For this review, take the finished solid that the model builds, in its own axes (mm). A direction names the side the tool comes from. Round coordinates to 2 decimals unless told otherwise and drop trailing zeros. Write each loop counter-clockwise with the first axis right and the second up, starting at its lowest first coordinate (ties: lowest second). Pieces come first, ordered by that corner, then holes. Notation, with made-up numbers: (15.5, 45) - (51.5, 45) arc R24 cw to (51.5, 57) - close; hole circle Ø5 at (47.25, -8). An arc over 180 degrees is marked (long way). Answer in a Markdown table with one row per item. Add a question column.
from build123d import *

# Parameters (mm, degrees)
SKETCH2_W         = 80
SKETCH2_H         = 60
FLOOR_2P4_DEPTH   = 2.4
WALLS_2P4_START   = 2.4
SKETCH3_W         = 80
SKETCH3_H         = 60
SKETCH3_W_2       = 75.2
SKETCH3_H_2       = 55.2
WALLS_2P4_DEPTH   = 33.6
CATCH_LEFT_START  = 21
SKETCH4_W         = 0.8
SKETCH4_H         = 12
CATCH_LEFT_DEPTH  = 2
CATCH_RIGHT_START = 21
SKETCH5_W         = 0.8
SKETCH5_H         = 12
CATCH_RIGHT_DEPTH = 2


with BuildPart() as part:
    # Sketch2 → Floor_2p4 (new body)
    with BuildSketch(Plane.XY):
        Rectangle(SKETCH2_W, SKETCH2_H)
    extrude(amount=FLOOR_2P4_DEPTH)

    # Sketch3 → Walls_2p4 (add)
    with BuildSketch(Plane.XY.offset(WALLS_2P4_START)):
        Rectangle(SKETCH3_W, SKETCH3_H)
        Rectangle(SKETCH3_W_2, SKETCH3_H_2, mode=Mode.SUBTRACT)
    extrude(amount=WALLS_2P4_DEPTH)

    # Sketch4 → Catch_left (add)
    with BuildSketch(Plane.XY.offset(CATCH_LEFT_START)):
        with Locations((-37.2, 0)):
            Rectangle(SKETCH4_W, SKETCH4_H)
    extrude(amount=CATCH_LEFT_DEPTH)

    # Sketch5 → Catch_right (add)
    with BuildSketch(Plane.XY.offset(CATCH_RIGHT_START)):
        with Locations((37.2, 0)):
            Rectangle(SKETCH5_W, SKETCH5_H)
    extrude(amount=CATCH_RIGHT_DEPTH)


solid = part.part
Q1. Draft analysis for pull direction Y (two halves, no side actions). For faces 4 (the face through (-40, 0, 18)), 5 (the face through (-1, 30, 18)), 6 (the face through (36.8, 0, 22)), state which applies: released by +Y, released by -Y, zero draft, split by the parting line, or undercut.
Q2. Tool access review of faces 1 (the face through (-1, -27.6, 19)), 2 (the face through (-37.6, 0, 19)), 3 (the face through (-3, -29, 36)): name each direction out of +Z, -Z, +X, -X, +Y, -Y from which nothing blocks a thin tool from reaching the whole face with its end or side.
Q3. Add section A-A on z = 13. State the section outline as (x, y) points, then the cut area to 3 significant figures.
Q4. Add section B-B on x = 19.5. State the section outline as (y, z) points, then the cut area to 3 significant figures.
Q5. To check wall thickness, follow probe 1 along Y at (x, z) = (-24.5, 26); probe 2 along X at (y, z) = (-22.5, 18.5); probe 3 along Z at (x, y) = (0.5, -5). State the ranges of each line that lie inside material, in increasing order.
Q6. Add section C-C on y = -24. State the section outline as (x, z) points.
Q7. Insertion check: pin 1 Ø1.5 at (x, y) = (13.5, -2.5) entering from +Z; pin 2 Ø0.9 at (x, y) = (-37, 1) entering from +Z. Each pin has a flat end and moves straight along its axis. Give the tip position at first contact, or say it passes through.
Answer sheet:
| question | item | result |
|---|---|---|
| 1 | face 4 | zero draft |
| 1 | face 5 | released by +Y |
| 1 | face 6 | undercut |
| 2 | face 1 | +Z |
| 2 | face 2 | none |
| 2 | face 3 | +Z, +X, -X, +Y, -Y |
| 3 | outline | (-40, -30) - (40, -30) - (40, 30) - (-40, 30) - close; hole (-37.6, -27.6) - (37.6, -27.6) - (37.6, 27.6) - (-37.6, 27.6) - close |
| 3 | area | 649 mm² |
| 4 | outline | (-30, 0) - (30, 0) - (30, 36) - (27.6, 36) - (27.6, 2.4) - (-27.6, 2.4) - (-27.6, 36) - (-30, 36) - close |
| 4 | area | 305 mm² |
| 5 | probe 1 | y = -30 to -27.6, 27.6 to 30 |
| 5 | probe 2 | x = -40 to -37.6, 37.6 to 40 |
| 5 | probe 3 | z = 0 to 2.4 |
| 6 | outline | (-40, 0) - (40, 0) - (40, 36) - (37.6, 36) - (37.6, 2.4) - (-37.6, 2.4) - (-37.6, 36) - (-40, 36) - close |
| 7 | pin 1 | stops at z = 2.4 |
| 7 | pin 2 | stops at z = 23 |
